Could you check a few things on this model? Use its own coordinates, in mm. Face numbers are marked on the shaded views. A direction names the side the tool comes from. Coordinates: 2 decimals unless noted, no trailing zeros. Loops run counter-clockwise (first coordinate to the right, second up) from the corner with the lowest first, then second, coordinate; pieces in that order, holes last.
1) Imagine slicing it at D-D on x = 10.19. Please give me the cut outline in (y, z) (3 decimals), plus the area to 3 significant figures.
2) Will these pins go through, and if not, where does the flat tip stop? P1, Ø2, axis at x = 24.5, y = 8.5, coming from the -Z side (3 decimals); P2, Ø1, axis at x = -17.5, z = -4.5, coming from the +Y side.
3) Imagine slicing it at C-C on y = 13. Please give me the cut outline in (x, z) (3 decimals), plus the area to 3 significant figures.
4) Imagine slicing it at B-B on y = 5. Please give me the cut outline in (x, z) (3 decimals), plus the area to 3 significant figures.
5) For the marked faces 4 and 5, which set-ups out of +Z, -Z, +X, -X, +Y, -Y let a thin tool reach every point of the face, with its end or its side?
6) Thinking about a two-plate mould opening in X: for the marked faces 1, 2 and 3, which applies, released by +X, released by -X, zero draft, split by the parting line, or undercut?
7) Imagine slicing it at A-A on x = -24.24. Please give me the cut outline in (y, z) (3 decimals), plus the area to 3 significant figures.
8) If I drill on line 1 along Y through (x, z) = (-24.24, 21.85); line 2 along X through (y, z) = (9.5, 19.5); line 3 along Z through (x, y) = (21.5, 9.25) (3 decimals), over which ranges is the centre line in solid material (lowest first)?
```python
from build123d import *

# Parameters (mm, degrees)
SKETCH1_W           = 54.98
SKETCH1_H           = 41.35
BOSS_EXTRUDE1_DEPTH = 3
SKETCH2_W           = 6.5
SKETCH2_H           = 5.65
SKETCH2_W_2         = 6.65
BOSS_EXTRUDE2_DEPTH = 20
SKETCH3_R           = 4.9
BOSS_EXTRUDE3_DEPTH = 15
CUT_EXTRUDE1_REACH  = 68.783
SKETCH4_R           = 2.6


with BuildPart() as part:
    # Sketch1 → Boss-Extrude1 (new body)
    with BuildSketch(Plane(origin=(0, 0, 0), x_dir=(1, 0, 0), z_dir=(0, 1, 0))):
        with Locations((0, -3)):
            Rectangle(SKETCH1_W, SKETCH1_H)
    extrude(amount=BOSS_EXTRUDE1_DEPTH)

    # Sketch2 → Boss-Extrude2 (add)
    with BuildSketch(Plane(origin=(0, 3, 0), x_dir=(1, 0, 0), z_dir=(0, 1, 0))):
        with Locations((-24.24, -20.85)):
            Rectangle(SKETCH2_W, SKETCH2_H)
        with Locations((24.165, -20.85)):
            Rectangle(SKETCH2_W_2, SKETCH2_H)
        Polygon((-27.49, 17.675), (27.49, 17.675), (27.49, 7.675), (24.49, 7.675), (24.49, 14.675), (-20.49, 14.675), (-20.49, 7.675), (-27.49, 7.675), align=None)
    extrude(amount=BOSS_EXTRUDE2_DEPTH)

    # Sketch3 → Boss-Extrude3 (add)
    with BuildSketch(Plane(origin=(0, 0, -17.675), x_dir=(-1, 0, 0), z_dir=(0, 0, -1))):
        with Locations((-10.19, 13)):
            Circle(SKETCH3_R)
    extrude(amount=BOSS_EXTRUDE3_DEPTH)

    # Sketch4 → Cut-Extrude1 (cut, up to next)
    with BuildSketch(Plane.XY.offset(23.675), mode=Mode.PRIVATE) as cut_extrude1_sk1:
        with Locations((-24.24, 17.5)):
            Circle(SKETCH4_R)
    cut_extrude1_tool1 = extrude(cut_extrude1_sk1.sketch, amount=-CUT_EXTRUDE1_REACH, mode=Mode.PRIVATE) & part.part
    # Sketch4 → Cut-Extrude1 (cut, up to next)
    with BuildSketch(Plane.XY.offset(23.675), mode=Mode.PRIVATE) as cut_extrude1_sk2:
        with Locations((-24.24, 8.5)):
            Circle(SKETCH4_R)
    cut_extrude1_tool2 = extrude(cut_extrude1_sk2.sketch, amount=-CUT_EXTRUDE1_REACH, mode=Mode.PRIVATE) & part.part
    # Sketch4 → Cut-Extrude1 (cut, up to next)
    with BuildSketch(Plane.XY.offset(23.675), mode=Mode.PRIVATE) as cut_extrude1_sk3:
        with Locations((24.24, 17.5)):
            Circle(SKETCH4_R)
    cut_extrude1_tool3 = extrude(cut_extrude1_sk3.sketch, amount=-CUT_EXTRUDE1_REACH, mode=Mode.PRIVATE) & part.part
    # Sketch4 → Cut-Extrude1 (cut, up to next)
    with BuildSketch(Plane.XY.offset(23.675), mode=Mode.PRIVATE) as cut_extrude1_sk4:
        with Locations((24.24, 8.5)):
            Circle(SKETCH4_R)
    cut_extrude1_tool4 = extrude(cut_extrude1_sk4.sketch, amount=-CUT_EXTRUDE1_REACH, mode=Mode.PRIVATE) & part.part
    add(cut_extrude1_tool1.solids().sort_by_distance((-24.24, 17.5, 23.675))[0], mode=Mode.SUBTRACT)
    add(cut_extrude1_tool2.solids().sort_by_distance((-24.24, 8.5, 23.675))[0], mode=Mode.SUBTRACT)
    add(cut_extrude1_tool3.solids().sort_by_distance((24.24, 17.5, 23.675))[0], mode=Mode.SUBTRACT)
    add(cut_extrude1_tool4.solids().sort_by_distance((24.24, 8.5, 23.675))[0], mode=Mode.SUBTRACT)


solid = part.part
```
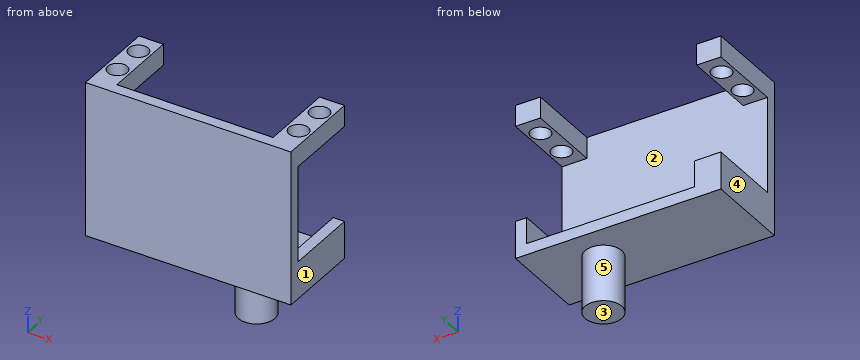
Filled in:
1. outline: (0, -17.675) - (8.1, -17.675) - (8.1, -32.675) - (17.9, -32.675) - (17.9, -17.675) - (23, -17.675) - (23, -14.675) - (3, -14.675) - (3, 23.675) - (0, 23.675) - close
1. area: 331 mm2
2. P1: stops at z = -17.675
2. P2: stops at y = 3
3. outline: (-27.49, -17.675) - (5.29, -17.675) - (5.29, -32.675) - (15.09, -32.675) - (15.09, -17.675) - (27.49, -17.675) - (27.49, -7.675) - (24.49, -7.675) - (24.49, -14.675) - (-20.49, -14.675) - (-20.49, -7.675) - (-27.49, -7.675) - close; (-27.49, 18.025) - (-20.99, 18.025) - (-20.99, 23.675) - (-27.49, 23.675) - close; (20.84, 18.025) - (27.49, 18.025) - (27.49, 23.675) - (20.84, 23.675) - close
3. area: 456 mm2
4. outline: (-27.49, -17.675) - (27.49, -17.675) - (27.49, -7.675) - (24.49, -7.675) - (24.49, -14.675) - (-20.49, -14.675) - (-20.49, -7.675) - (-27.49, -7.675) - close; (-27.49, 18.025) - (-20.99, 18.025) - (-20.99, 23.675) - (-27.49, 23.675) - close; (20.84, 18.025) - (27.49, 18.025) - (27.49, 23.675) - (20.84, 23.675) - close
4. area: 309 mm2
5. face 4: +Z, -Z, -X, +Y, -Y
5. face 5: -Z
6. face 1: released by +X
6. face 2: undercut
6. face 3: zero draft
7. outline: (0, -17.675) - (23, -17.675) - (23, -7.675) - (3, -7.675) - (3, 18.025) - (5.9, 18.025) - (5.9, 23.675) - (0, 23.675) - close; (11.1, 18.025) - (14.9, 18.025) - (14.9, 23.675) - (11.1, 23.675) - close; (20.1, 18.025) - (23, 18.025) - (23, 23.675) - (20.1, 23.675) - close
7. area: 378 mm2
8. line 1: y = 0 to 5.9, 11.1 to 14.9, 20.1 to 23
8. line 2: x = -27.49 to -26.64, -21.84 to -20.99, 20.84 to 21.84, 26.64 to 27.49
8. line 3: z = -17.675 to -14.675, 18.025 to 23.675
